Work out the finished part from the listing and answer in its coordinate system (mm). A direction names the side the tool comes from. Round coordinates to 2 decimals unless told otherwise and drop trailing zeros. Order: outer loops, then holes, each group sorted by start corner. A loop starts at its lowest first (then second) coordinate and runs counter-clockwise, first axis right, second up.
Autodesk Inventor part; units mm, degrees
ref_plane "YZ Plane" through (0, 0, 0) normal (1, 0, 0) x (0, 1, 0)
ref_plane "XZ Plane" through (0, 0, 0) normal (0, 1, 0) x (-1, 0, 0)
ref_plane "XY Plane" through (0, 0, 0) normal (0, 0, 1) x (1, 0, 0)
sketch "スケッチ1" plane through (0, 0, 0) normal (0, 1, 0) x (-1, 0, 0)
  line L0 (-350, 350) -> (350, 350)
  line L1 (350, 350) -> (350, -350)
  line L2 (350, -350) -> (-350, -350)
  line L3 (-350, -350) -> (-350, 350)
  line L4 (-350, 350) -> (350, -350) construction
  line L5 (350, 350) -> (-350, -350) construction
  point P0 (0, 0)
  dimension "d0" = 700
  dimension "d1" = 700
extrude "押し出し1" add sketch "スケッチ1" along normal blind 20
sketch "スケッチ2" plane through (350, 0, 350) normal (1, 0, 0) x (0, 0, -1)
  line L0 (0, 0) -> (0, 20)
  line L1 (0, 0) -> (700, 0)
  line L2 (700, 0) -> (700, -340)
  line L3 (700, -340) -> (0, -340)
  line L4 (0, -340) -> (0, 0)
  point P0 (350, 0)
  dimension "d4" = 700
  dimension "d5" = 340
extrude "押し出し2" add sketch "スケッチ2" against normal blind 20
sketch "スケッチ3" plane through (-350, 0, -350) normal (-1, 0, 0) x (0, 0, 1)
  line L0 (0, 20) -> (0, -340)
  line L1 (0, -340) -> (700, -340)
  line L2 (0, 0) -> (700, 0)
  line L3 (700, 0) -> (700, -340)
  line L4 (700, -340) -> (0, -340)
  line L5 (0, -340) -> (0, 0)
  point P0 (350, 0)
extrude "押し出し3" add sketch "スケッチ3" against normal blind 20
sketch "スケッチ4" plane through (-350, 20, 350) normal (0, 0, 1) x (1, 0, 0)
  line L0 (20, -20) -> (20, -360)
  line L1 (680, -360) -> (680, -20)
  line L2 (20, -20) -> (680, -20)
  line L3 (680, -20) -> (680, -360)
  line L4 (680, -360) -> (20, -360)
  line L5 (20, -360) -> (20, -20)
  point P0 (350, -20)
extrude "押し出し4" add sketch "スケッチ4" against normal blind 20
properties part number "こたつ"
Item 1: Find section A-A (z = -293.5). Write down the section's boundary in (x, y).
Item 2: Find section C-C (x = 4). Write down the section's boundary in (y, z).
Item 3: Find section B-B (y = -92.5). Write down the section's boundary in (x, z).
Item 4: Find the intervals of material crossed by line 1 along X through (y, z) = (-140.5, 149); line 2 along Y through (x, z) = (-251, -196); line 3 along Z through (x, y) = (-48.5, -15), in increasing order.
Item 5: A tool of negligible diameter and unlimited length cuts with its end or side. For faces 1 (the face through (5, 0, -5)), 2 (the face through (-2, 1, -350)), from which of +Z, -Z, +X, -X, +Y, -Y can it reach the whole face along a straight path? Write none if from no direction.
Item 6: For a pull along X with two mould halves and no side action, classify faces 3 (the face through (-5, -168, 330)), 4 (the face through (-350, -157, -5)), 5 (the face through (-5, -157, 350)) as released by +X, released by -X, zero draft, split by the parting line, or undercut.
Item 7: Given pin 1 (1.5 mm diameter, centred on x = 165.5, z = 275, fed in from -Y); pin 2 (4 mm diameter, centred on x = -195.5, y = -148, fed in from -Z), each flat-ended and moving along its own axis, determine where each tip first touches the part or whether it passes through.
Model answer:
1. outline: (-350, -340) - (-330, -340) - (-330, 0) - (330, 0) - (330, -340) - (350, -340) - (350, 20) - (-350, 20) - close
2. outline: (-340, 330) - (0, 330) - (0, -350) - (20, -350) - (20, 350) - (-340, 350) - close
3. outline: (-350, -350) - (-330, -350) - (-330, 330) - (330, 330) - (330, -350) - (350, -350) - (350, 350) - (-350, 350) - close
4. line 1: x = -350 to -330, 330 to 350
4. line 2: y = 0 to 20
4. line 3: z = 330 to 350
5. face 1: -Z, -Y
5. face 2: -Z, +X, -X, +Y, -Y
6. face 3: undercut
6. face 4: released by -X
6. face 5: zero draft
7. pin 1: stops at y = 0
7. pin 2: stops at z = 330
